The listing builds one solid part. Answer for the finished solid, in the listing's coordinates (mm). A direction names the side the tool comes from. Round coordinates to 2 decimals unless told otherwise and drop trailing zeros. Loops run counter-clockwise (first coordinate to the right, second up) from the corner with the lowest first, then second, coordinate; pieces in that order, holes last. Notation, with made-up numbers: (8.25, -3.75) -> (26.25, -3.75) arc R32 ccw to (26.25, 28.25) -> close; hole circle Ø10 at (-35, 80.25). An arc over 180 degrees is marked (long way). Write each question's results on one line, items separated by ' | '. Start each with the question number.
(1) The part is cut by section A-A (x = 0). Determine the outline of the cut face in (y, z), plus the area to 3 significant figures.
(2) Determine the mould class of faces 4 (the face through (5.22, 2.96, 1.23)), 5 (the face through (0, -6, 1)), 6 (the face through (3, 0, 1)) for opening direction X: released by +X, released by -X, zero draft, split by the parting line, or undercut.
(3) The part is cut by section C-C (x = -5.25). Determine the outline of the cut face in (y, z), plus the area to 3 significant figures.
(4) The part is cut by section B-B (z = 48.5). Determine the outline of the cut face in (x, y).
(5) Straight lines are drawn through the part: probe 1 along Y at (x, z) = (0, 0.6); probe 2 along Y at (x, z) = (-2, 38); probe 3 along Z at (x, y) = (-2, 4.5). For each, find the intervals that lie inside material, in ascending order.
(6) For faces 1 (the face through (-3, 3, 2.5)), 2 (the face through (0, 0, 2)), 3 (the face through (0, 0, 52.5)), determine the directions among +Z, -Z, +X, -X, +Y, -Y from which every point of the face is accessible in a straight line to the end or side of a thin tool.
(7) Flat-ended cylindrical pins translate along their axes: pin 1 (4 mm diameter, centred on y = 4, z = 13, fed in from -X); pin 2 (8 mm diameter, centred on x = -2.5, z = 31, fed in from +Y); pin 3 (5 mm diameter, centred on x = -1.5, y = -1, fed in from -Z); pin 4 (1 mm diameter, centred on y = 3, z = 18.5, fed in from -X). Find the tip coordinate at first contact, or state that the pin passes through.
Autodesk Inventor part; units mm, degrees
ref_plane "YZ Plane" through (0, 0, 0) normal (1, 0, 0) x (0, 1, 0)
ref_plane "XZ Plane" through (0, 0, 0) normal (0, 1, 0) x (-1, 0, 0)
ref_plane "XY Plane" through (0, 0, 0) normal (0, 0, 1) x (1, 0, 0)
sketch "Skizze1" plane through (0, 0, 0) normal (0, 0, 1) x (1, 0, 0)
  circle A0 centre (0, 0) radius 6
  dimension "d0" = 12
extrude "Extrusion1" add sketch "Skizze1" along normal blind 2.5
sketch "Skizze2" plane through (0, 0, 2.5) normal (0, 0, 1) x (1, 0, 0)
  circle A0 centre (0, 0) radius 4
  dimension "d3" = 8
extrude "Extrusion2" add sketch "Skizze2" along normal blind 50
sketch "Skizze3" plane through (0, 0, 0) normal (0, 0, -1) x (-1, 0, 0)
  circle A0 centre (0, 0) radius 3
  dimension "d6" = 6
extrude "Extrusion3" cut sketch "Skizze3" against normal blind 2
sketch "Skizze4" plane through (0, 0, 0) normal (0, 0, -1) x (-1, 0, 0)
  line L0 (3.4641, 6) -> (6.9282, 0)
  line L1 (6.9282, 0) -> (3.4641, -6)
  line L2 (3.4641, -6) -> (-3.4641, -6)
  line L3 (-3.4641, -6) -> (-6.9282, 0)
  line L4 (-6.9282, 0) -> (-3.4641, 6)
  line L5 (-3.4641, 6) -> (3.4641, 6)
  circle A0 centre (0, 0) radius 3
  dimension "d9" = 12
extrude "Extrusion4" add sketch "Skizze4" against normal up to surface (2.5 mm away)
chamfer "Fase1" distance 0.5 angle 45 1 edges at (-4, 0, 52.5)
thread "Gewinde1"
properties part number "Bolzen" material "Messing, weicher Gelbton"
Checked values:
1) outline: (-6, 0) -> (-3, 0) -> (-3, 2) -> (3, 2) -> (3, 0) -> (6, 0) -> (6, 2.5) -> (4, 2.5) -> (4, 52) -> (3.5, 52.5) -> (-3.5, 52.5) -> (-4, 52) -> (-4, 2.5) -> (-6, 2.5) -> close | area: 418 mm2
2) face 4: released by +X | face 5: zero draft | face 6: undercut
3) outline: (-2.91, 0) -> (2.91, 0) -> (2.91, 2.5) -> (-2.91, 2.5) -> close | area: 14.5 mm2
4) outline: circle Ø8 at (0, 0)
5) probe 1: y = -6 to -3, 3 to 6 | probe 2: y = -3.46 to 3.46 | probe 3: z = 0 to 2.5
6) face 1: +Z | face 2: -Z | face 3: +Z, +X, -X, +Y, -Y
7) pin 1: stops at x = -3.46 | pin 2: stops at y = 4 | pin 3: stops at z = 0 | pin 4: stops at x = -3.12
